from build123d import *

# Parameters (mm, degrees)
SKETCH1_W           = 90
SKETCH1_H           = 90
SKETCH1_R           = 3.55
SKETCH1_W_2         = 66
SKETCH1_H_2         = 65.290786417
BOSS_EXTRUDE1_DEPTH = 10
CUT_EXTRUDE1_REACH  = 103.119
SKETCH2_R           = 1.5
SKETCH3_R           = 2
CUT_EXTRUDE2_DEPTH  = 90
SKETCH4_R           = 2
CUT_EXTRUDE3_DEPTH  = 90


with BuildPart() as part:
    # Sketch1 → Boss-Extrude1 (new body)
    with BuildSketch(Plane.XY):
        Rectangle(SKETCH1_W, SKETCH1_H)
        with Locations((-38.185, 38.182532328)):
            Circle(SKETCH1_R, mode=Mode.SUBTRACT)
        with Locations(Location((38.185, 38.182532328, 0), (0, 0, 180))):
            Circle(SKETCH1_R, mode=Mode.SUBTRACT)
        with Locations((38.185, -38.182532328)):
            Circle(SKETCH1_R, mode=Mode.SUBTRACT)
        with Locations(Location((-38.185, -38.182532328, 0), (0, 0, 180))):
            Circle(SKETCH1_R, mode=Mode.SUBTRACT)
        with Locations((0, 0.354606792)):
            Rectangle(SKETCH1_W_2, SKETCH1_H_2, mode=Mode.SUBTRACT)
    extrude(amount=BOSS_EXTRUDE1_DEPTH)

    # Sketch2 → Cut-Extrude1 (cut, up to next)
    with BuildSketch(Plane.XZ.offset(45), mode=Mode.PRIVATE) as cut_extrude1_sk1:
        with Locations((-38.89, 5)):
            Circle(SKETCH2_R)
    cut_extrude1_tool1 = extrude(cut_extrude1_sk1.sketch, amount=-CUT_EXTRUDE1_REACH, mode=Mode.PRIVATE) & part.part
    # Sketch2 → Cut-Extrude1 (cut, up to next)
    with BuildSketch(Plane.XZ.offset(45), mode=Mode.PRIVATE) as cut_extrude1_sk2:
        with Locations((38.89, 5)):
            Circle(SKETCH2_R)
    cut_extrude1_tool2 = extrude(cut_extrude1_sk2.sketch, amount=-CUT_EXTRUDE1_REACH, mode=Mode.PRIVATE) & part.part
    cut_extrude1_1 = cut_extrude1_tool1.solids().sort_by_distance((-38.89, -45, 5))[0]
    add(cut_extrude1_1, mode=Mode.SUBTRACT)
    cut_extrude1_2 = cut_extrude1_tool2.solids().sort_by_distance((38.89, -45, 5))[0]
    add(cut_extrude1_2, mode=Mode.SUBTRACT)
    cut_extrude1 = cut_extrude1_1 + cut_extrude1_2  # Cut-Extrude1 as one shape, for the pattern or mirror that repeats it

    # Mirror1: Cut-Extrude1 across plane
    add(cut_extrude1.mirror(Plane.ZX), mode=Mode.SUBTRACT)

    # Sketch3 → Cut-Extrude2 (cut)
    with BuildSketch(Plane.XZ.offset(45)):
        with Locations((-25, 5)):
            Circle(SKETCH3_R)
        with Locations((25, 5)):
            Circle(SKETCH3_R)
    extrude(amount=-CUT_EXTRUDE2_DEPTH, mode=Mode.SUBTRACT)

    # Sketch4 → Cut-Extrude3 (cut)
    with BuildSketch(Plane.ZY.offset(45)):
        with Locations(Location((5, 25, 0), (0, 0, 270))):
            Circle(SKETCH4_R)
        with Locations(Location((5, -25, 0), (0, 0, 270))):
            Circle(SKETCH4_R)
    extrude(amount=-CUT_EXTRUDE3_DEPTH, mode=Mode.SUBTRACT)


solid = part.part
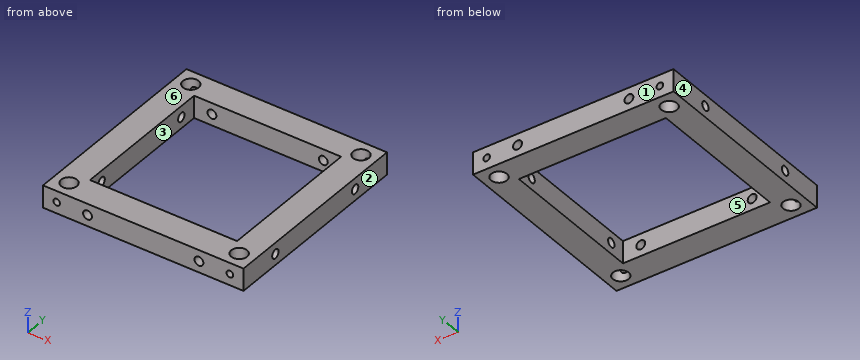
Can you work these out from the model? Positions are in its coordinate system, mm. Face numbers are marked on the shaded views. A direction names the side the tool comes from. Round coordinates to 2 decimals unless told otherwise and drop trailing zeros. Write each loop counter-clockwise with the first axis right and the second up, starting at its lowest first coordinate (ties: lowest second). Pieces come first, ordered by that corner, then holes. Notation, with made-up numbers: (58.5, 17) -> (80.5, 17) arc R18 ccw to (80.5, 51) -> close; hole circle Ø9 at (-34, -1.5). An arc over 180 degrees is marked (long way). Use one line per item in the form item = value. Start each with the question number.
Q1. We'd pull the mould along X, two halves only. Please class the marked faces 1, 2, 3 and 4: +X half, -X half, draft (parallel to the pull), parting line (faces both ways), or undercut.
Q2. Imagine slicing it at A-A (y = -16). Please give me the cut outline in (x, z), then the cut area to 3 significant figures.
Q3. Imagine slicing it at B-B (x = -25). Please give me the cut outline in (y, z), then the cut area to 3 significant figures.
Q4. I'm going to push flat-ended pins straight in: P1, Ø9, axis at x = 38.18, y = -38.18, coming from the -Z side; P2, Ø2.5, axis at x = 38.89, z = 5, coming from the -Y side. Where does each tip first touch, or does it pass through?
Q5. Which directions (+Z, -Z, +X, -X, +Y, -Y) give clear straight access to the entire face, cutting with the end or side of a thin tool? Please do the marked faces 5 and 6.
Q6. If I drill on probe 1 along X at (y, z) = (-5.5, 8); probe 2 along Y at (x, z) = (-19.5, 8); probe 3 along Z at (x, y) = (-25, 41.25), over which ranges is the centre line in solid material (lowest first)? Write a range as [from, to].
Q7. Imagine slicing it at C-C (x = 31). Please give me the cut outline in (y, z), then the cut area to 3 significant figures.
Q8. Imagine slicing it at D-D (y = 25). Please give me the cut outline in (x, z), then the cut area to 3 significant figures.
Worked out:
q1.face_1 = draft
q1.face_2 = +X half
q1.face_3 = undercut
q1.face_4 = -X half
q2.outline = (-45, 0) -> (-33, 0) -> (-33, 10) -> (-45, 10) -> close; (33, 0) -> (45, 0) -> (45, 10) -> (33, 10) -> close
q2.area = 240 mm^2
q3.outline = (-45, 0) -> (-32.29, 0) -> (-32.29, 3) -> (-45, 3) -> close; (-45, 7) -> (-32.29, 7) -> (-32.29, 10) -> (-45, 10) -> close; (33, 0) -> (45, 0) -> (45, 3) -> (33, 3) -> close; (33, 7) -> (45, 7) -> (45, 10) -> (33, 10) -> close
q3.area = 148 mm^2
q4.P1 = 0
q4.P2 = -35.22
q5.face_5 = +Z, -Z
q5.face_6 = +Z, +X, -X, +Y, -Y
q6.probe_1 = [-45, -33], [33, 45]
q6.probe_2 = [-45, -32.29], [33, 45]
q6.probe_3 = [0, 3], [7, 10]
q7.outline = (-45, 0) -> (-32.29, 0) -> (-32.29, 10) -> (-45, 10) -> close; (33, 0) -> (45, 0) -> (45, 10) -> (33, 10) -> close
q7.area = 247 mm^2
q8.outline = (-45, 0) -> (-33, 0) -> (-33, 3) -> (-45, 3) -> close; (-45, 7) -> (-33, 7) -> (-33, 10) -> (-45, 10) -> close; (33, 0) -> (45, 0) -> (45, 3) -> (33, 3) -> close; (33, 7) -> (45, 7) -> (45, 10) -> (33, 10) -> close
q8.area = 144 mm^2
